Verification items for the finished model (mm, model axes). Face numbers are marked on the shaded views. A direction names the side the tool comes from. Give positions to 0.01 mm unless a question says otherwise; leave off trailing zeros. Write each loop counter-clockwise with the first axis right and the second up, starting at its lowest first coordinate (ties: lowest second). Pieces come first, ordered by that corner, then holes. Notation, with made-up numbers: (72, -40) - (84, -40) arc R16 ccw to (84, -18) - close; hole circle Ø4 at (47, 36.25). An arc over 180 degrees is marked (long way). Answer as a JSON object with one key per item and string values. Group by question number.
Item 1: Sectioned sample at B-B, the plane y = 4.5. Record the boundary of the cut face in (x, z), and give its area (3 significant figures).
Item 2: Go/stop test with flat-tipped pins: pin 1 (5.5 mm diameter, centred on x = -49, z = 1, fed in from +Y); pin 2 (12 mm diameter, centred on x = -41.5, y = -41, fed in from +Z); pin 3 (1.5 mm diameter, centred on y = -49, z = -0.5, fed in from +X); pin 4 (6 mm diameter, centred on y = -50, z = 0, fed in from -X). Record where each tip stops, or that it passes through.
Item 3: Sectioned sample at D-D, the plane z = 7.5. Record the boundary of the cut face in (x, y), and give its area (3 significant figures).
Item 4: Tool access check on the marked faces 1 and 2. Record the directions out of +Z, -Z, +X, -X, +Y, -Y that give a thin tool (end or side, any length) a straight path to the whole face; none if there is none.
Item 5: Scan lines: line 1 along Z through (x, y) = (5.25, -50); line 2 along Y through (x, z) = (16.5, 0.75); line 3 along X through (y, z) = (15.5, 1.5). Record each from-to range of solid material in increasing order. Write a range as [from, to].
Item 6: Sectioned sample at A-A, the plane z = 0. Record the boundary of the cut face in (x, y).
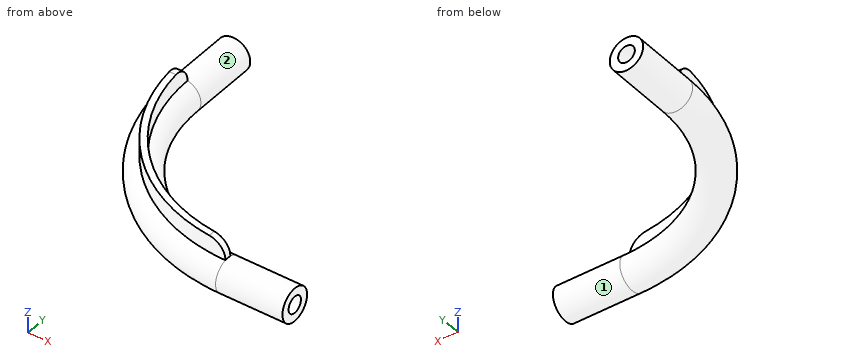
```python
from build123d import *

# Parameters (mm, degrees)
SKETCH_4_R      = 5
REVOLVE_1_ANGLE = 90
SKETCH_5_R      = 5
SKETCH_5_R_2    = 2.5
EXTRUDE_4_DEPTH = 20
SKETCH_6_R      = 5
SKETCH_6_R_2    = 2.5
EXTRUDE_5_DEPTH = 20
EXTRUDE_6_DEPTH = 10
FILLET_1_R      = 5


with BuildPart() as part:
    # 草圖4 → 旋轉1 (revolve)
    with BuildSketch(Plane(origin=(0, 0, 0), x_dir=(1, 0, 0), z_dir=(0, 1, 0))):
        with Locations((-50, 0)):
            Circle(SKETCH_4_R)
    revolve(axis=Axis((0, 0, -3.474942085), (0, 0, 1)), revolution_arc=REVOLVE_1_ANGLE)

    # 草圖5 → 填料-伸長4 (add)
    with BuildSketch(Plane(origin=(0, 0, 0), x_dir=(0, 0, -1), z_dir=(1, 0, 0))):
        with Locations(Location((0, -50, 0), (0, 0, 270))):
            Circle(SKETCH_5_R)
        with Locations(Location((0, -50, 0), (0, 0, 90))):
            Circle(SKETCH_5_R_2, mode=Mode.SUBTRACT)
    extrude(amount=EXTRUDE_4_DEPTH)

    # 草圖6 → 填料-伸長5 (add)
    with BuildSketch(Plane(origin=(0, 0, 0), x_dir=(1, 0, 0), z_dir=(0, 1, 0))):
        with Locations(Location((-50, 0, 0), (0, 0, 180))):
            Circle(SKETCH_6_R)
        with Locations(Location((-50, 0, 0), (0, 0, 270))):
            Circle(SKETCH_6_R_2, mode=Mode.SUBTRACT)
    extrude(amount=EXTRUDE_5_DEPTH)

    # 草圖7 → 填料-伸長6 (add)
    with BuildSketch(Plane.XY):
        with BuildLine():
            Line((-49, 0), (-51, 0))
            ThreePointArc((-51, 0), (-36.062445841, -36.062445841), (0, -51))
            Line((0, -51), (0, -49))
            ThreePointArc((0, -49), (-34.648232278, -34.648232278), (-49, 0))
        make_face()
    extrude(amount=EXTRUDE_6_DEPTH)

    # 圓角1
    fillet_1_edges = [part.edges().sort_by_distance(p)[0] for p in [
        (-50, 0, 10),
        (0, -50, 10),
    ]]
    fillet(fillet_1_edges, radius=FILLET_1_R - 0.0001)  # a hair under: the kernel refuses the full size


solid = part.part
```
Geometry check:
{
 "1": {"outline": "circle Ø10 at (-50, 0); hole circle Ø5 at (-50, 0)", "area": "58.9 mm^2"},
 "2": {"pin 1": "y = 20", "pin 2": "z = 4.42", "pin 3": "x = 0", "pin 4": "x = -28.57"},
 "3": {"outline": "(-51, -0.67) arc R51 ccw to (-0.67, -51) - (-0.67, -49) arc R49 cw to (-49, -0.67) - close", "area": "154 mm^2"},
 "4": {"face 1": "+X", "face 2": "+Y"},
 "5": {"line 1": "[-5, -2.5], [2.5, 5]", "line 2": "[-54.94, -52.38], [-47.62, -45.06]", "line 3": "[-54.77, -52], [-48, -45.23]"},
 "6": {"outline": "(-55, 0) arc R55 ccw to (0, -55) - (20, -55) - (20, -52.5) - (0, -52.5) - (0, -47.5) - (20, -47.5) - (20, -45) - (0, -45) arc R45 cw to (-45, 0) - (-45, 20) - (-47.5, 20) - (-47.5, 0) - (-52.5, 0) - (-52.5, 20) - (-55, 20) - close"}
}
